```python
from build123d import *

# Parameters (mm, degrees)
ESBO_O2_R                = 15
RESSALTO_EXTRUS_O1_DEPTH = 20
FUROS_GUIA_COM_10_0MM1_D = 10.4
CORTE_EXTRUS_O1_DEPTH    = 30.154759474
FILETE1_R                = 5


with BuildPart() as part:
    # Esboço2 → Ressalto-extrusão1 (new body)
    with BuildSketch(Plane(origin=(0, 0, 0), x_dir=(1, 0, 0), z_dir=(0, 1, 0))):
        with Locations(Location((0, 0, 0), (0, 0, 270))):
            Circle(ESBO_O2_R)
    extrude(amount=RESSALTO_EXTRUS_O1_DEPTH)

    # Furos-guia com Ø10.0mm1 (through all)
    with Locations(Plane(origin=(0, 20, 0), x_dir=(1, 0, 0), z_dir=(0, 1, 0))):
        with Locations((0, 0)):
            Hole(FUROS_GUIA_COM_10_0MM1_D / 2)

    # Esboço6 → Corte-extrusão1 (cut, through all)
    with BuildSketch(Plane(origin=(0, 20, 0), x_dir=(1, 0, 0), z_dir=(0, 1, 0))):
        with BuildLine():
            Line((-1.65, 4.931277725), (-1.65, 6.531277725))
            Line((-1.65, 6.531277725), (1.65, 6.531277725))
            Line((1.65, 6.531277725), (1.65, 4.931277725))
            ThreePointArc((1.65, 4.931277725), (0, 5.189536775), (-1.65, 4.931277725))
        make_face()
    extrude(amount=-CORTE_EXTRUS_O1_DEPTH, mode=Mode.SUBTRACT)

    # Esboço7 → Corte-Revolução1 (revolve, cut)
    with BuildSketch(Plane.XY, mode=Mode.PRIVATE) as corte_revolu_o1_sk:
        Polygon((-15, 18), (-15, 2), (-7, 4.911761874), (-7, 15.088238126), align=None)
    revolve(corte_revolu_o1_sk.sketch.rotate(Axis((0, 0, 0), (0, 1, 0)), 270), axis=Axis((0, 0, 0), (0, 1, 0)), mode=Mode.SUBTRACT)

    # Filete1
    filete1_edges = [part.edges().sort_by_distance(p)[0] for p in [
        (0, 15.088238126, 7),
        (0, 4.911761874, 7),
    ]]
    fillet(filete1_edges, radius=FILETE1_R)


solid = part.part
```
Verification items for the finished model (mm, model axes). A direction names the side the tool comes from. Round coordinates to 2 decimals unless told otherwise and drop trailing zeros. Put each result on its own line as item: value. Start each with the question number.
(1) Tool access check on faces 1 (the face through (-1.65, 10, -6)), 2 (the face through (-8.87, 3.63, -5.65)), 3 (the face through (0, 20, 6)). Record the directions out of +Z, -Z, +X, -X, +Y, -Y that give a thin tool (end or side, any length) a straight path to the whole face; none if there is none.
(2) Depth check by flat-ended pin: pin 1 Ø1 at (x, y) = (-0.5, 8) entering from +Z; pin 2 Ø1.5 at (y, z) = (14, -3) entering from -X; pin 3 Ø0.5 at (y, z) = (10, -6) entering from -X; pin 4 Ø5 at (x, z) = (3.5, 11.5) entering from -Y. Enter the tip coordinate at first touch or a pass-through.
(3) Material ranges on line 1 along X through (y, z) = (10.25, 0); line 2 along Y through (x, z) = (-2.5, 13); line 3 along Y through (x, z) = (-4, 12.5), recorded low to high.
(4) Draft check along Y on faces 4 (the face through (0.66, 18.986, -14.985)), 5 (the face through (0, 0, 6)), 6 (the face through (-3.179, 16.393, -10.096)). Enter one of: +Y half, -Y half, draft (parallel to the pull), parting line (faces both ways), or undercut.
Completed:
1. face 1: +Y, -Y
1. face 2: none
1. face 3: +Z, -Z, +X, -X, +Y
2. pin 1: stops at z = 7.07
2. pin 2: stops at x = -7.61
2. pin 3: stops at x = -3.99
2. pin 4: stops at y = 0
3. line 1: x = -7 to -5.2, 5.2 to 7
3. line 2: y = 0 to 2.64, 17.36 to 20
3. line 3: y = 0 to 2.68, 17.32 to 20
4. face 4: draft
4. face 5: -Y half
4. face 6: undercut
